```python
from build123d import *

# Parameters (mm, degrees)
SKETCH1_W               = 10
SKETCH1_H               = 95
BOSS_EXTRUDE1_DEPTH     = 40
SKETCH4_W               = 10
SKETCH4_H               = 80
BOSS_EXTRUDE3_DEPTH     = 70
SKETCH10_R              = 11
SKETCH10_R_2            = 1.6
CUT_EXTRUDE1_DEPTH      = 10
SKETCH2_R               = 11
SKETCH2_R_2             = 1.55
SKETCH2_R_3             = 2.05
CUT_EXTRUDE2_DEPTH      = 10
BOSS_EXTRUDE4_DEPTH     = 5
SKETCH15_R              = 3.25
CUT_EXTRUDE3_DEPTH      = 5
CROQUIS1_W              = 50
CROQUIS1_H              = 22
CROQUIS1_R              = 9.72345
SALIENTE_EXTRUIR1_DEPTH = 10
CROQUIS2_R              = 3.1
CORTAR_EXTRUIR1_DEPTH   = 7
REDONDEO1_R             = 10


with BuildPart() as part:
    # Sketch1 → Boss-Extrude1 (new, symmetric)
    with BuildSketch(Plane(origin=(0, 0, 0), x_dir=(1, 0, 0), z_dir=(0, 1, 0))):
        with Locations((-5, -1.933942264)):
            Rectangle(SKETCH1_W, SKETCH1_H)
    extrude(amount=BOSS_EXTRUDE1_DEPTH, both=True)

    # Sketch4 → Boss-Extrude3 (add)
    with BuildSketch(Plane(origin=(0, 0, 0), x_dir=(0, 0, -1), z_dir=(1, 0, 0))):
        with Locations((40.566057736, 0)):
            Rectangle(SKETCH4_W, SKETCH4_H)
    extrude(amount=BOSS_EXTRUDE3_DEPTH)

    # Sketch10 → Cut-Extrude1 (cut)
    with BuildSketch(Plane(origin=(0, 0, -45.566057736), x_dir=(-1, 0, 0), z_dir=(0, 0, -1))):
        with Locations((-35, 0)):
            Circle(SKETCH10_R)
        with Locations((-19.5, 15.5)):
            Circle(SKETCH10_R_2)
        with Locations((-50.5, 15.5)):
            Circle(SKETCH10_R_2)
        with Locations((-19.5, -15.5)):
            Circle(SKETCH10_R_2)
        with Locations((-50.5, -15.5)):
            Circle(SKETCH10_R_2)
    extrude(amount=-CUT_EXTRUDE1_DEPTH, mode=Mode.SUBTRACT)

    # Sketch2 → Cut-Extrude2 (cut)
    with BuildSketch(Plane.ZY.offset(10)):
        with Locations((-0.566057736, 0)):
            Circle(SKETCH2_R)
        with Locations((-15.591169934, -15.5)):
            Circle(SKETCH2_R_2)
        with Locations((-6.916057736, -19.05)):
            Circle(SKETCH2_R_3)
        with Locations((-15.591169934, 15.5)):
            Circle(SKETCH2_R_2)
        with Locations((-6.916057736, 19.05)):
            Circle(SKETCH2_R_3)
        with Locations((5.783942264, 19.05)):
            Circle(SKETCH2_R_3)
        with Locations((14.459054462, 15.5)):
            Circle(SKETCH2_R_2)
        with Locations((14.459054462, -15.5)):
            Circle(SKETCH2_R_2)
        with Locations((5.783942264, -19.05)):
            Circle(SKETCH2_R_3)
    extrude(amount=-CUT_EXTRUDE2_DEPTH, mode=Mode.SUBTRACT)

    # Sketch14 → Boss-Extrude4 (add)
    with BuildSketch(Plane.XY.offset(49.433942264)):
        with BuildLine():
            Line((-15, -17.5), (-10, -17.5))
            Line((-10, -17.5), (-10, -7.5))
            Line((-10, -7.5), (-15, -7.5))
            ThreePointArc((-15, -7.5), (-20, -12.5), (-15, -17.5))
        make_face()
        with BuildLine():
            Line((-15, 7.5), (-10, 7.5))
            Line((-10, 7.5), (-10, 17.5))
            Line((-10, 17.5), (-15, 17.5))
            ThreePointArc((-15, 17.5), (-20, 12.5), (-15, 7.5))
        make_face()
    extrude(amount=-BOSS_EXTRUDE4_DEPTH)

    # Sketch15 → Cut-Extrude3 (cut)
    with BuildSketch(Plane(origin=(0, 0, 44.433942264), x_dir=(-1, 0, 0), z_dir=(0, 0, -1))):
        with Locations((15, -12.5)):
            Circle(SKETCH15_R)
        with Locations((15, 12.5)):
            Circle(SKETCH15_R)
    extrude(amount=-CUT_EXTRUDE3_DEPTH, mode=Mode.SUBTRACT)

    # Croquis1 → Saliente-Extruir1 (add)
    with BuildSketch(Plane(origin=(0, 40, 0), x_dir=(1, 0, 0), z_dir=(0, 1, 0))):
        with Locations((25, 0.566057736)):
            Rectangle(CROQUIS1_W, CROQUIS1_H)
        with Locations(Location((35, 0.566057736, 0), (0, 0, 270))):
            Circle(CROQUIS1_R, mode=Mode.SUBTRACT)
    extrude(amount=-SALIENTE_EXTRUIR1_DEPTH)

    # Croquis2 → Cortar-Extruir1 (cut)
    with BuildSketch(Plane(origin=(70, 0, 0), x_dir=(0, 0, -1), z_dir=(1, 0, 0))):
        with Locations((40.566057736, 30)):
            Circle(CROQUIS2_R)
        with Locations((40.566057736, -30)):
            Circle(CROQUIS2_R)
    extrude(amount=-CORTAR_EXTRUIR1_DEPTH, mode=Mode.SUBTRACT)

    # Redondeo1
    redondeo1_edges = [part.edges().sort_by_distance(p)[0] for p in [
        (0, 0, -35.566057736),
        (0, 35, -11.566057736),
        (0, 35, 10.433942264),
    ]]
    fillet(redondeo1_edges, radius=REDONDEO1_R)


solid = part.part
```
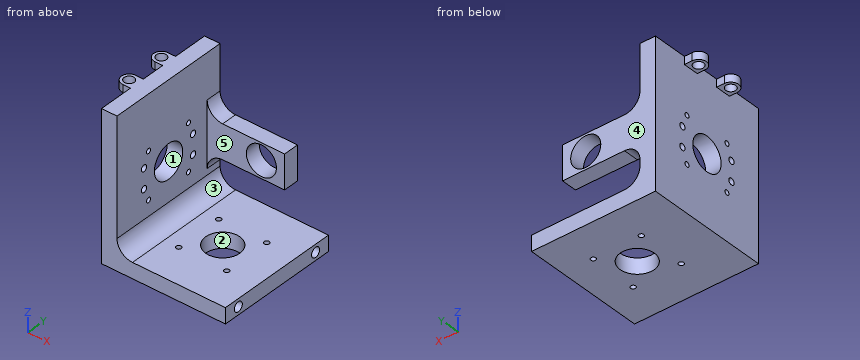
Input: part model. Units: mm. Frame: model coordinates. Face numbers are marked on the shaded views. A direction names the side the tool comes from. Round coordinates to 2 decimals unless told otherwise and drop trailing zeros. Loops run counter-clockwise (first coordinate to the right, second up) from the corner with the lowest first, then second, coordinate; pieces in that order, holes last.
1) Pull-direction query (X, two-part tool) for the marked faces 1, 2 and 3; classes: released by +X, released by -X, zero draft, split by the parting line, or undercut.
Ans:
face 1: zero draft
face 2: undercut
face 3: released by +X
2) Material intervals for line 1 (Z direction, x = -3, y = -19); line 2 (Y direction, x = -15, z = 46.8); line 3 (Z direction, x = 19, y = 31.5), sorted ascending.
Ans:
line 1: z = -45.57 to -8.97, -4.87 to 3.73, 7.83 to 49.43
line 2: y = -17.5 to -15.75, -9.25 to -7.5, 7.5 to 9.25, 15.75 to 17.5
line 3: z = -45.57 to -35.57, -11.57 to 10.43
3) Section query A-A on y = 0. Return the cut outline in (x, z).
Ans:
outline: (-10, -45.57) - (24, -45.57) - (24, -35.57) - (10, -35.57) arc R10 cw to (0, -25.57) - (0, -11.57) - (-10, -11.57) - close; (-10, 10.43) - (0, 10.43) - (0, 49.43) - (-10, 49.43) - close; (46, -45.57) - (70, -45.57) - (70, -35.57) - (46, -35.57) - close
4) Section query C-C on x = -2. Count the separate pieces of the cut face and the enclosed holes in it, plus the area to 3 significant figures.
Ans:
separate pieces: 1
enclosed holes: 9
area: 7,140 mm2
5) Section query B-B on x = 35. Return the cut outline in (y, z).
Ans:
outline: (-40, -45.57) - (-11, -45.57) - (-11, -35.57) - (-40, -35.57) - close; (11, -45.57) - (40, -45.57) - (40, -35.57) - (11, -35.57) - close; (30, -11.57) - (40, -11.57) - (40, -10.29) - (30, -10.29) - close; (30, 9.16) - (40, 9.16) - (40, 10.43) - (30, 10.43) - close
6) Pin query (flat end, axial travel): pin 1 (3 mm diameter, centred on y = 37, z = 1.5, fed in from +X); pin 2 (6 mm diameter, centred on x = 53, y = -2.5, fed in from +Z); pin 3 (4 mm diameter, centred on x = -12.5, z = 47.5, fed in from -Y); pin 4 (3.5 mm diameter, centred on x = 50.5, y = -15.5, fed in from -Z). Return the tip coordinate at first contact, or that it passes through.
Ans:
pin 1: stops at x = 50
pin 2: stops at z = -35.57
pin 3: stops at y = -17.5
pin 4: stops at z = -45.57
7) Set-up query: the marked faces 4 and 5. Return all of +Z, -Z, +X, -X, +Y, -Y with unobstructed straight access to the full face (end or side cutting, diameter ignored); none if empty.
Ans:
face 4: +Z, -Z, +X, -X, +Y
face 5: +Z, +X, -Y
8) Section query D-D on y = -12.5. Return the cut outline in (x, z).
Ans:
outline: (-20, 44.43) - (-18.25, 44.43) - (-18.25, 49.43) - (-20, 49.43) - close; (-11.75, 44.43) - (-10, 44.43) - (-10, -45.57) - (70, -45.57) - (70, -35.57) - (10, -35.57) arc R10 cw to (0, -25.57) - (0, 49.43) - (-11.75, 49.43) - close
